Input: dimensioned drawing with shaded views. Units: mm. Origin: part minimum x, y, z. A direction names the side the tool comes from. Give positions to 0.01 mm unless a question says otherwise; leave off trailing zeros. Write each loop counter-clockwise with the first axis right and the second up, starting at its lowest first coordinate (ties: lowest second). Pieces come first, ordered by that corner, then holes. Notation, with made-up numbers: (63, 74) - (103, 74) arc R21 cw to (103, 111) - close; hole circle Ø1 at (80, 86.5). An arc over 180 degrees is marked (long way). Answer as a JSON object with one key per item and string values. Group by question number.
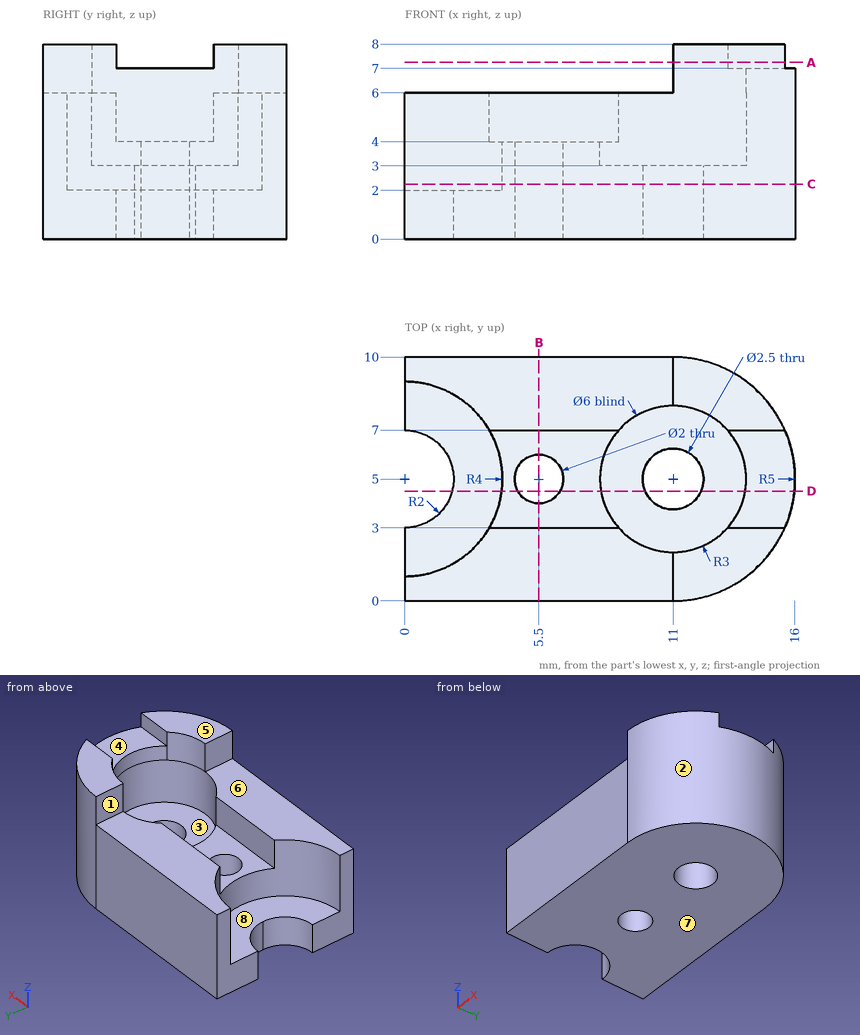
1) Line query: line 1 along X through (y, z) = (5, 1.4); line 2 along X through (y, z) = (3, 3.25); line 3 along Y through (x, z) = (5.5, 2.6). Output: solid intervals per line, ascending. Write a range as from..to.
2) Reachability of the marked faces 4, 5, 6, 7 and 8 from +Z, -Z, +X, -X, +Y, -Y: full face, straight path, thin tool, end or side. Return the list, or none.
3) Pin query (flat end, axial travel): P1, Ø1, axis at y = 1, z = 7.5, coming from the -X side; P2, Ø1.8, axis at x = 5.5, y = 5, coming from the +Z side; P3, Ø4, axis at x = 8.5, y = 8.5, coming from the +Z side; P4, Ø3, axis at x = 11, y = 5, coming from the +Z side. Return the tip coordinate at first contact, or that it passes through.
4) Cut plane A-A on z = 7.25. Return the cut outline in (x, y).
5) Cut plane D-D on y = 4.5. Return the cut outline in (x, z).
6) Cut plane C-C on z = 2.25. Return the cut outline in (x, y), and give its area (3 significant figures).
7) Cut plane B-B on x = 5.5. Return the cut outline in (y, z), and give its area (3 significant figures).
8) Mould query, pull axis Y, two halves, no side actions, for the marked faces 1, 2 and 3. Classes: +Y half, -Y half, draft (parallel to the pull), parting line (faces both ways), or undercut.
Filled in:
{
 "1": {"line 1": "x = 2..4.5, 6.5..9.75, 12.25..16", "line 2": "x = 3.46..8.76, 13.24..15.58", "line 3": "y = 0..4, 6..10"},
 "2": {"face 4": "+Z, +X, -X", "face 5": "+Z, +X, -X, +Y, -Y", "face 6": "+Z, -X, +Y, -Y", "face 7": "-Z, +X, -X, +Y, -Y", "face 8": "+Z, -X"},
 "3": {"P1": "stops at x = 11", "P2": "passes through", "P3": "stops at z = 6", "P4": "stops at z = 3"},
 "4": {"outline": "(11, 0) arc R5 ccw to (15.58, 3) - (13.24, 3) arc R3 cw to (11, 2) - close; (11, 8) arc R3 cw to (13.24, 7) - (15.58, 7) arc R5 ccw to (11, 10) - close"},
 "5": {"outline": "(1.94, 0) - (4.63, 0) - (4.63, 4) - (3.97, 4) - (3.97, 2) - (1.94, 2) - close; (6.37, 0) - (9.85, 0) - (9.85, 3) - (8.04, 3) - (8.04, 4) - (6.37, 4) - close; (12.15, 0) - (15.97, 0) - (15.97, 7) - (13.96, 7) - (13.96, 3) - (12.15, 3) - close"},
 "6": {"outline": "(0, 0) - (11, 0) arc R5 ccw to (11, 10) - (0, 10) - (0, 9) arc R4 cw to (0, 1) - close; hole circle Ø2 at (5.5, 5); hole circle Ø2.5 at (11, 5)", "area": "116 mm²"},
 "7": {"outline": "(0, 0) - (4, 0) - (4, 4) - (3, 4) - (3, 6) - (0, 6) - close; (6, 0) - (10, 0) - (10, 6) - (7, 6) - (7, 4) - (6, 4) - close", "area": "44.0 mm²"},
 "8": {"face 1": "draft", "face 2": "parting line", "face 3": "undercut"}
}
